```python
from build123d import *

# Parameters (mm, degrees)
EXTRUDE_4_DEPTH     = 65
CUT_EXTRUDE_2_DEPTH = 24.5
CUT_EXTRUDE_3_DEPTH = 24.5
CUT_EXTRUDE_5_REACH = 108.333
SKETCH_11_R         = 1.5
SKETCH_11_W         = 60.605178709
SKETCH_11_H         = 18
CUT_EXTRUDE_4_REACH = 108.359
SKETCH_8_R          = 1.5


with BuildPart() as part:
    # 草图1 → 凸台-拉伸4 (new body)
    with BuildSketch(Plane.XY):
        Polygon((0, 0), (0, 3), (7, 3), (69.785178709, 19.823237932), (74.785178709, 19.823237932), (74.785178709, 3), (81.785178709, 3), (81.785178709, 0), align=None)
    extrude(amount=EXTRUDE_4_DEPTH)

    # 草图9 → 切除-拉伸2 (cut)
    with BuildSketch(Plane.XY.offset(65)):
        Polygon((65.110092512, 16.5), (10.995355803, 2), (71.610092512, 2), (71.610092512, 16.5), align=None)
    extrude(amount=-CUT_EXTRUDE_2_DEPTH, mode=Mode.SUBTRACT)

    # 草图10 → 切除-拉伸3 (cut)
    with BuildSketch(Plane(origin=(0, 0, 0), x_dir=(-1, 0, 0), z_dir=(0, 0, -1))):
        Polygon((-71.610092512, 2), (-10.995355803, 2), (-65.110092512, 16.5), (-71.610092512, 16.5), align=None)
    extrude(amount=-CUT_EXTRUDE_3_DEPTH, mode=Mode.SUBTRACT)

    # 草图11 → 切除-拉伸5 (cut, up to next)
    with BuildSketch(Plane.XZ, mode=Mode.PRIVATE) as cut_extrude_5_sk1:
        with Locations(Location((3.892589354, 60.5, 0), (0, 0, 270))):
            Circle(SKETCH_11_R)
    cut_extrude_5_tool1 = extrude(cut_extrude_5_sk1.sketch, amount=-CUT_EXTRUDE_5_REACH, mode=Mode.PRIVATE) & part.part
    # 草图11 → 切除-拉伸5 (cut, up to next)
    with BuildSketch(Plane.XZ, mode=Mode.PRIVATE) as cut_extrude_5_sk2:
        with Locations(Location((77.892589354, 60.5, 0), (0, 0, 270))):
            Circle(SKETCH_11_R)
    cut_extrude_5_tool2 = extrude(cut_extrude_5_sk2.sketch, amount=-CUT_EXTRUDE_5_REACH, mode=Mode.PRIVATE) & part.part
    # 草图11 → 切除-拉伸5 (cut, up to next)
    with BuildSketch(Plane.XZ, mode=Mode.PRIVATE) as cut_extrude_5_sk3:
        with Locations(Location((77.892589354, 4.5, 0), (0, 0, 270))):
            Circle(SKETCH_11_R)
    cut_extrude_5_tool3 = extrude(cut_extrude_5_sk3.sketch, amount=-CUT_EXTRUDE_5_REACH, mode=Mode.PRIVATE) & part.part
    # 草图11 → 切除-拉伸5 (cut, up to next)
    with BuildSketch(Plane.XZ, mode=Mode.PRIVATE) as cut_extrude_5_sk4:
        with Locations(Location((3.892589354, 4.5, 0), (0, 0, 270))):
            Circle(SKETCH_11_R)
    cut_extrude_5_tool4 = extrude(cut_extrude_5_sk4.sketch, amount=-CUT_EXTRUDE_5_REACH, mode=Mode.PRIVATE) & part.part
    # 草图11 → 切除-拉伸5 (cut, up to next)
    with BuildSketch(Plane.XZ, mode=Mode.PRIVATE) as cut_extrude_5_sk5:
        with Locations((41.302589355, 49.5)):
            Rectangle(SKETCH_11_W, SKETCH_11_H)
    cut_extrude_5_tool5 = extrude(cut_extrude_5_sk5.sketch, amount=-CUT_EXTRUDE_5_REACH, mode=Mode.PRIVATE) & part.part
    # 草图11 → 切除-拉伸5 (cut, up to next)
    with BuildSketch(Plane.XZ, mode=Mode.PRIVATE) as cut_extrude_5_sk6:
        with Locations((41.302589355, 15.5)):
            Rectangle(SKETCH_11_W, SKETCH_11_H)
    cut_extrude_5_tool6 = extrude(cut_extrude_5_sk6.sketch, amount=-CUT_EXTRUDE_5_REACH, mode=Mode.PRIVATE) & part.part
    add(cut_extrude_5_tool1.solids().sort_by_distance((3.892589, 0, 60.5))[0], mode=Mode.SUBTRACT)
    add(cut_extrude_5_tool2.solids().sort_by_distance((77.892589, 0, 60.5))[0], mode=Mode.SUBTRACT)
    add(cut_extrude_5_tool3.solids().sort_by_distance((77.892589, 0, 4.5))[0], mode=Mode.SUBTRACT)
    add(cut_extrude_5_tool4.solids().sort_by_distance((3.892589, 0, 4.5))[0], mode=Mode.SUBTRACT)
    add(cut_extrude_5_tool5.solids().sort_by_distance((41.302589, 0, 49.5))[0], mode=Mode.SUBTRACT)
    add(cut_extrude_5_tool6.solids().sort_by_distance((41.302589, 0, 15.5))[0], mode=Mode.SUBTRACT)

    # 草图8 → 切除-拉伸4 (cut, up to next)
    with BuildSketch(Plane(origin=(-0.281088913, 1.049038106, 0), x_dir=(0.9659258262890681, 0.25881904510252157, 0), z_dir=(-0.25881904510252157, 0.9659258262890681, 0)), mode=Mode.PRIVATE) as cut_extrude_4_sk1:
        with Locations(Location((16.037937919, -14.5, 0), (0, 0, 180))):
            Circle(SKETCH_8_R)
    cut_extrude_4_tool1 = extrude(cut_extrude_4_sk1.sketch, amount=-CUT_EXTRUDE_4_REACH, mode=Mode.PRIVATE) & part.part
    # 草图8 → 切除-拉伸4 (cut, up to next)
    with BuildSketch(Plane(origin=(-0.281088913, 1.049038106, 0), x_dir=(0.9659258262890681, 0.25881904510252157, 0), z_dir=(-0.25881904510252157, 0.9659258262890681, 0)), mode=Mode.PRIVATE) as cut_extrude_4_sk2:
        with Locations(Location((64.037937919, -14.5, 0), (0, 0, 180))):
            Circle(SKETCH_8_R)
    cut_extrude_4_tool2 = extrude(cut_extrude_4_sk2.sketch, amount=-CUT_EXTRUDE_4_REACH, mode=Mode.PRIVATE) & part.part
    # 草图8 → 切除-拉伸4 (cut, up to next)
    with BuildSketch(Plane(origin=(-0.281088913, 1.049038106, 0), x_dir=(0.9659258262890681, 0.25881904510252157, 0), z_dir=(-0.25881904510252157, 0.9659258262890681, 0)), mode=Mode.PRIVATE) as cut_extrude_4_sk3:
        with Locations(Location((64.037937919, -50.5, 0), (0, 0, 180))):
            Circle(SKETCH_8_R)
    cut_extrude_4_tool3 = extrude(cut_extrude_4_sk3.sketch, amount=-CUT_EXTRUDE_4_REACH, mode=Mode.PRIVATE) & part.part
    # 草图8 → 切除-拉伸4 (cut, up to next)
    with BuildSketch(Plane(origin=(-0.281088913, 1.049038106, 0), x_dir=(0.9659258262890681, 0.25881904510252157, 0), z_dir=(-0.25881904510252157, 0.9659258262890681, 0)), mode=Mode.PRIVATE) as cut_extrude_4_sk4:
        with Locations(Location((16.037937919, -50.5, 0), (0, 0, 180))):
            Circle(SKETCH_8_R)
    cut_extrude_4_tool4 = extrude(cut_extrude_4_sk4.sketch, amount=-CUT_EXTRUDE_4_REACH, mode=Mode.PRIVATE) & part.part
    add(cut_extrude_4_tool1.solids().sort_by_distance((15.21037, 5.199962, 14.5))[0], mode=Mode.SUBTRACT)
    add(cut_extrude_4_tool2.solids().sort_by_distance((61.574809, 17.623276, 14.5))[0], mode=Mode.SUBTRACT)
    add(cut_extrude_4_tool3.solids().sort_by_distance((61.574809, 17.623276, 50.5))[0], mode=Mode.SUBTRACT)
    add(cut_extrude_4_tool4.solids().sort_by_distance((15.21037, 5.199962, 50.5))[0], mode=Mode.SUBTRACT)


solid = part.part
```
For this review, take the finished solid that the model builds, in its own axes (mm). A direction names the side the tool comes from. Coordinates: 2 decimals unless noted, no trailing zeros. Write each loop counter-clockwise with the first axis right and the second up, starting at its lowest first coordinate (ties: lowest second). Pieces come first, ordered by that corner, then holes. Notation, with made-up numbers: (-8.75, -20.5) - (41.25, -20.5) arc R20 ccw to (41.25, 0.5) - close; hole circle Ø2 at (26.5, -16.5). An arc over 180 degrees is marked (long way). Put each result on its own line as item: value.
1. Mouldability with a two-part tool opening along X and no side actions: class faces 1 (the flat face through (81.785, 2, 32)), 2 (the flat face through (0, 1, 32)), 3 (the flat face through (41, 2, 63)) as released by +X, released by -X, zero draft, split by the parting line, or undercut.
Values found:
face 1: released by +X
face 2: released by -X
face 3: undercut
2. For pin 1 (5 mm diameter, centred on x = 68.5, z = 47.5, fed in from -Y); pin 2 (19.5 mm diameter, centred on x = 48, z = 13, fed in from +Y); pin 3 (4 mm diameter, centred on x = 3.89, z = 60.5, fed in from +Y), all flat-tipped, find the tip position at first contact; note any pin that passes through.
Values found:
pin 1: y = 16.5
pin 2: y = 16.6
pin 3: y = 3
3. Add section A-A, the plane z = 4.5. Give the boundary of the cut face in (x, y).
Values found:
outline: (0, 0) - (2.39, 0) - (2.39, 3) - (0, 3) - close; (5.39, 0) - (76.39, 0) - (76.39, 3) - (74.79, 3) - (74.79, 19.82) - (69.79, 19.82) - (7, 3) - (5.39, 3) - close; (79.39, 0) - (81.79, 0) - (81.79, 3) - (79.39, 3) - close; hole (11, 2) - (71.61, 2) - (71.61, 16.5) - (65.11, 16.5) - close
4. Wall thickness on probe 1 along X at (y, z) = (1.6, 4.5); probe 2 along Z at (x, y) = (70, 6.5); probe 3 along Y at (x, z) = (30, 42): over which ranges is each line inside the solid? List them lowest first.
Values found:
probe 1: 0 to 2.39, 5.39 to 76.39, 79.39 to 81.79
probe 2: 24.5 to 40.5
probe 3: 7.09 to 9.16
5. Add section D-D, the plane y = 9.5. Give the boundary of the cut face in (x, z).
Values found:
outline: (31.26, 0) - (38.99, 0) - (38.99, 24.5) - (71.61, 24.5) - (71.61, 0) - (74.79, 0) - (74.79, 65) - (71.61, 65) - (71.61, 40.5) - (38.99, 40.5) - (38.99, 65) - (31.26, 65) - close
6. Machinability: for faces 4 (the flat face through (71.61, 9, 12)), 5 (the flat face through (48, 6, 40.5)), 6 (the flat face through (68, 16.5, 53)), 7 (the flat face through (74.785, 12, 32)), which of the approach directions +Z, -Z, +X, -X, +Y, -Y give a long, thin tool a straight path to every point of the face, cutting with its end or side? Answer none if there is none.
Values found:
face 4: -Z
face 5: -Y
face 6: +Z
face 7: +Z, -Z, +X, +Y
7. Add section C-C, the plane x = 28. Give the boundary of the cut face in (y, z), then the cut area to 3 significant figures.
Values found:
outline: (0, 0) - (2, 0) - (2, 6.5) - (0, 6.5) - close; (0, 24.5) - (6.56, 24.5) - (6.56, 0) - (8.63, 0) - (8.63, 65) - (6.56, 65) - (6.56, 40.5) - (0, 40.5) - close; (0, 58.5) - (2, 58.5) - (2, 65) - (0, 65) - close
area: 265 mm²
